Can you work these out from the model? Positions are in its coordinate system, mm. A direction names the side the tool comes from. Give positions to 0.01 mm unless a question says otherwise; leave off trailing zeros. Loops run counter-clockwise (first coordinate to the right, second up) from the corner with the lowest first, then second, coordinate; pieces in that order, holes last. Notation, with made-up numbers: (62.5, 36) -> (119.5, 36) arc R14 ccw to (119.5, 51) -> close; hole circle Ø1 at (-21.75, -13). An arc over 180 degrees is marked (long way). Use CSV: the item, a comma, the result in double quotes.
from build123d import *

# Parameters (mm, degrees)
SKETCH1_W           = 40
SKETCH1_H           = 40
SKETCH1_W_2         = 36
SKETCH1_H_2         = 36
EXTRUDE_THIN1_DEPTH = 1216
SKETCH4_R           = 12.5
CUT_EXTRUDE2_DEPTH  = 10
SKETCH5_R           = 12.5
CUT_EXTRUDE3_DEPTH  = 10
SKETCH6_R           = 6
CUT_EXTRUDE4_DEPTH  = 10
SKETCH7_R           = 6
CUT_EXTRUDE5_DEPTH  = 10
LPATTERN2_COUNT     = 8
LPATTERN2_PITCH     = 152


with BuildPart() as part:
    # Sketch1 → Extrude-Thin1 (new body)
    with BuildSketch(Plane.XY):
        Rectangle(SKETCH1_W, SKETCH1_H)
        Rectangle(SKETCH1_W_2, SKETCH1_H_2, mode=Mode.SUBTRACT)
    extrude(amount=EXTRUDE_THIN1_DEPTH)

    # Sketch4 → Cut-Extrude2 (cut)
    with BuildSketch(Plane(origin=(20, 0, 0), x_dir=(0, 0, -1), z_dir=(1, 0, 0))):
        with Locations((-1140, -2)):
            Circle(SKETCH4_R)
    cut_extrude2 = extrude(amount=-CUT_EXTRUDE2_DEPTH, mode=Mode.SUBTRACT)

    # Sketch5 → Cut-Extrude3 (cut)
    with BuildSketch(Plane.XZ.offset(20)):
        with Locations((2, 1140)):
            Circle(SKETCH5_R)
    cut_extrude3 = extrude(amount=-CUT_EXTRUDE3_DEPTH, mode=Mode.SUBTRACT)

    # Sketch6 → Cut-Extrude4 (cut)
    with BuildSketch(Plane(origin=(-18, 0, 0), x_dir=(0, 0, -1), z_dir=(1, 0, 0))):
        with Locations((-1140, -2)):
            Circle(SKETCH6_R)
    cut_extrude4 = extrude(amount=-CUT_EXTRUDE4_DEPTH, mode=Mode.SUBTRACT)

    # Sketch7 → Cut-Extrude5 (cut)
    with BuildSketch(Plane(origin=(0, 20, 0), x_dir=(1, 0, 0), z_dir=(0, 1, 0))):
        with Locations(Location((2, -1140, 0), (0, 0, 180))):
            Circle(SKETCH7_R)
    cut_extrude5 = extrude(amount=-CUT_EXTRUDE5_DEPTH, mode=Mode.SUBTRACT)

    # LPattern2: Cut-Extrude2, Cut-Extrude3, Cut-Extrude4, Cut-Extrude5 ×8
    with Locations(*[(0, 0, -i * LPATTERN2_PITCH) for i in range(1, LPATTERN2_COUNT)]):
        add(cut_extrude2, mode=Mode.SUBTRACT)
        add(cut_extrude3, mode=Mode.SUBTRACT)
        add(cut_extrude4, mode=Mode.SUBTRACT)
        add(cut_extrude5, mode=Mode.SUBTRACT)


solid = part.part
(1) If we section it at A-A, the plane z = 576: Write out the boundary of the cut face in (x, y), then the cut area to 3 significant figures.
Answer sheet:
outline,"(-20, -20) -> (20, -20) -> (20, 20) -> (-20, 20) -> close; hole (-18, -18) -> (18, -18) -> (18, 18) -> (-18, 18) -> close"
area,"304 mm2"
(2) If I drill on L1, parallel to X at y = 15, z = 1101.5; L2, parallel to Y at x = -19, z = 988, over which ranges is the centre line in solid material (lowest first)? Write a range as from..to.
Answer sheet:
L1,"x = -20..-18, 18..20"
L2,"y = -20..-8, 4..20"
(3) We'd pull the mould along X, two halves only. Please class faces 4 (the face through (20, 0, 599)), 5 (the face through (19.014, -1.45, 544.488)), 6 (the face through (-0.71, -19.014, 975.797)): released by +X, released by -X, zero draft, split by the parting line, or undercut.
Answer sheet:
face 4,"released by +X"
face 5,"zero draft"
face 6,"undercut"
(4) Will these pins go through, and if not, where does the flat tip stop? pin 1 Ø9.5 at (y, z) = (-2, 684) entering from +X; pin 2 Ø15.5 at (x, z) = (2, 1140) entering from -Y.
Answer sheet:
pin 1,"passes through"
pin 2,"stops at y = 18"
(5) Which directions (+Z, -Z, +X, -X, +Y, -Y) give clear straight access to the entire face, cutting with the end or side of a thin tool? Please do faces 1 (the face through (13.923, -19.014, 79.755)), 2 (the face through (19.014, -1.45, 696.488)), 3 (the face through (0, 18, 599)).
Answer sheet:
face 1,"-Y"
face 2,"+X"
face 3,"+Z, -Z"
(6) If we section it at B-B, the plane y = -2: Give the number of separate pieces and of enclosed holes in the cut face, then the cut area to 3 significant figures.
Answer sheet:
separate pieces,"18"
enclosed holes,"0"
area,"4,270 mm2"
